Job drawing, mm, ordinate dimensions from the low corner. One solid piece. A direction names the side the tool comes from. Coordinates: 2 decimals unless noted, no trailing zeros. Write each loop counter-clockwise with the first axis right and the second up, starting at its lowest first coordinate (ties: lowest second). Pieces come first, ordered by that corner, then holes. Notation, with made-up numbers: M 23.5,34 L 68.5,34 A18 ccw 68.5,57 Z; hole C 26,75 d2. An arc over 180 degrees is marked long. Answer as CSV lines item,"result". Start each with the question number.
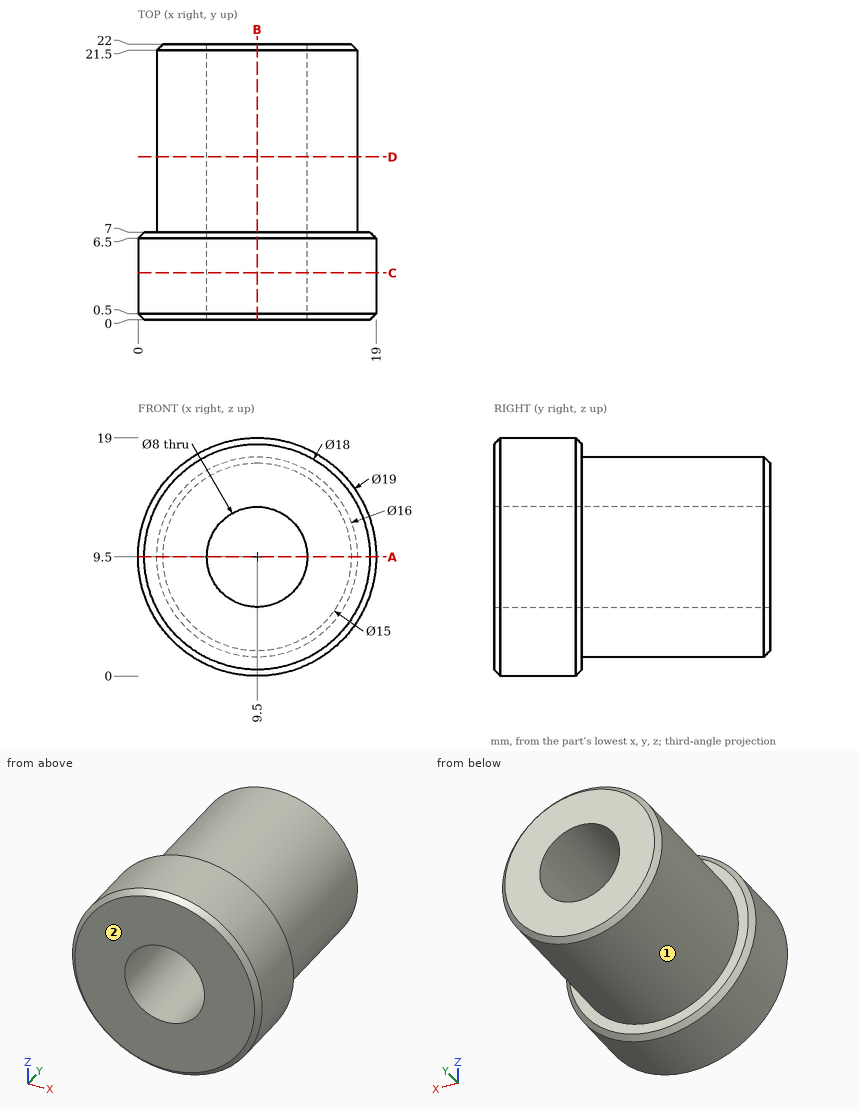
1) Band-saw the part on B-B, the plane x = 9.5. List the corners of the cut face in (y, z).
2) Tool access for the marked faces 1 and 2: list every direction of +Z, -Z, +X, -X, +Y, -Y with a clear straight run to the whole face (end or side of a thin tool).
3) Probe L1, parallel to X at y = 12.75, z = 9.5; L2, parallel to Z at x = 13, y = 9.5; L3, parallel to Z at x = 11, y = 11. List the from-to ranges inside material, lowest first. Write a range as [from, to].
4) Band-saw the part on D-D, the plane y = 13. List the corners of the cut face in (x, z).
5) Band-saw the part on C-C, the plane y = 3.75. List the corners of the cut face in (x, z).
6) Pin check, flat tips, straight feed: P1, Ø4, axis at x = 13, y = 17, coming from the +Z side; P2, Ø2, axis at x = 3, z = 17, coming from the -Y side; P3, Ø8, axis at y = 19.5, z = 7, coming from the +X side. Stop position of each tip, or through.
7) Band-saw the part on A-A, the plane z = 9.5. List the corners of the cut face in (x, y), plus the area to 3 significant figures.
Result sheet:
1,outline,"M 0,0.5 L 0.5,0 L 6.5,0 L 7,0.5 L 7,1.5 L 21.5,1.5 L 22,2 L 22,5.5 L 0,5.5 Z; M 0,13.5 L 22,13.5 L 22,17 L 21.5,17.5 L 7,17.5 L 7,18.5 L 6.5,19 L 0.5,19 L 0,18.5 Z"
2,face 1,"+Y"
2,face 2,"+Z, -Z, +X, -X, -Y"
3,L1,"x = [1.5, 5.5], [13.5, 17.5]"
3,L2,"z = [2.31, 7.56], [11.44, 16.69]"
3,L3,"z = [1.64, 5.79], [13.21, 17.36]"
4,outline,"C 9.5,9.5 d16; hole C 9.5,9.5 d8"
5,outline,"C 9.5,9.5 d19; hole C 9.5,9.5 d8"
6,P1,"stops at z = 17.36"
6,P2,"stops at y = 0"
6,P3,"stops at x = 17.5"
7,outline,"M 0,0.5 L 0.5,0 L 5.5,0 L 5.5,22 L 2,22 L 1.5,21.5 L 1.5,7 L 0.5,7 L 0,6.5 Z; M 13.5,0 L 18.5,0 L 19,0.5 L 19,6.5 L 18.5,7 L 17.5,7 L 17.5,21.5 L 17,22 L 13.5,22 Z"
7,area,"196 mm²"
